Here's how the part is built. I have some questions about the finished solid (model axes, mm). Round coordinates to 2 decimals unless told otherwise and drop trailing zeros. Write each loop counter-clockwise with the first axis right and the second up, starting at its lowest first coordinate (ties: lowest second). Pieces come first, ordered by that corner, then holes. Notation, with made-up numbers: (8, 68.5) -> (18, 68.5) arc R15 ccw to (18, 88.5) -> close; hole circle Ø4 at (-35, 18.25). An arc over 180 degrees is marked (long way). Put each result on its own line as item: value. Start each with the question number.
1. We'd pull the mould along X, two halves only. Please class faces 1 (the face through (0.534, -4.065, 10.34)), 2 (the face through (-4, 2, -0.9)), 3 (the face through (4.762, 1.974, -0.844)): +X half, -X half, draft (parallel to the pull), parting line (faces both ways), or undercut.
2. I need wall thicknesses on probe 1 along Y at (x, z) = (0, 15.5); probe 2 along Y at (x, z) = (-1.25, 15.75); probe 3 along X at (y, z) = (3.5, 7.25). Which ranges of each line are inside material? Lowest first, please. Write a range as from..to.
3. For pin 1 (1 mm diameter, centred on x = 1, y = -6, fed in from +Z); pin 2 (1 mm diameter, centred on x = 4.5, z = 17, fed in from -Y); pin 3 (3 mm diameter, centred on x = 6, y = -5, fed in from -Z), each with a flat end and sliding along its axis, tell me the tip position at first contact or that it passes through.
4. Suppose I cut it at C-C (z = 7.75). Please give me the cut outline in (x, y), then the cut area to 3 significant figures.
```python
from build123d import *
from OCP.BRepFilletAPI import BRepFilletAPI_MakeChamfer

# Parameters (mm, degrees)
SKETCH1_R           = 7.5
SKETCH1_R_2         = 4.1
BOSS_EXTRUDE1_DEPTH = 21
BOSS_EXTRUDE2_START = -0.9
SKETCH2_R           = 5
SKETCH2_R_2         = 4.1
BOSS_EXTRUDE2_DEPTH = 22.8
CHAMFER1_SIZE       = 0.9
CHAMFER1_SIZE_2     = 2.472729678


with BuildPart() as part:
    # Sketch1 → Boss-Extrude1 (new body)
    with BuildSketch(Plane.XY):
        with Locations(Location((0, 0, 0), (0, 0, 180))):
            Circle(SKETCH1_R)
        with Locations(Location((0, 0, 0), (0, 0, 180))):
            Circle(SKETCH1_R_2, mode=Mode.SUBTRACT)
    extrude(amount=BOSS_EXTRUDE1_DEPTH)

    # Sketch2 → Boss-Extrude2 (add)
    with BuildSketch(Plane.XY.offset(BOSS_EXTRUDE2_START)):
        Circle(SKETCH2_R)
        with Locations(Location((0, 0, 0), (0, 0, 180))):
            Circle(SKETCH2_R_2, mode=Mode.SUBTRACT)
    extrude(amount=BOSS_EXTRUDE2_DEPTH)

    # Chamfer1
    chamfer1_edges_1 = [part.edges().sort_by_distance(p)[0] for p in [
        (-5, 0, 0),
    ]]
    chamfer1_side_1 = [part.faces().sort_by_distance(p)[0] for p in [
        (-5, 0, -0.018),
    ]]
    chamfer1_edges_2 = [part.edges().sort_by_distance(p)[0] for p in [
        (-5, 0, 21),
    ]]
    chamfer1_side_2 = [part.faces().sort_by_distance(p)[0] for p in [
        (-5.018, 0, 21),
    ]]
    chamfer1 = BRepFilletAPI_MakeChamfer(part.part.solid().wrapped)
    for e in chamfer1_edges_1:
        chamfer1.Add(CHAMFER1_SIZE - 0.0001, CHAMFER1_SIZE_2 - 0.0001, e.wrapped, chamfer1_side_1[0].wrapped)
    for e in chamfer1_edges_2:
        chamfer1.Add(CHAMFER1_SIZE_2 - 0.0001, CHAMFER1_SIZE - 0.0001, e.wrapped, chamfer1_side_2[0].wrapped)
    add(Compound.cast(chamfer1.Shape()), mode=Mode.REPLACE)  # a hair under: the kernel refuses the full size


solid = part.part
```
Verdict:
1. face 1: undercut
1. face 2: draft
1. face 3: parting line
2. probe 1: y = -7.5..-4.1, 4.1..7.5
2. probe 2: y = -7.4..-3.9, 3.9..7.4
2. probe 3: x = -6.63..-2.14, 2.14..6.63
3. pin 1: stops at z = 21.69
3. pin 2: stops at y = -6.34
3. pin 3: stops at z = -0.42
4. outline: circle Ø15 at (0, 0); hole circle Ø8.2 at (0, 0)
4. area: 124 mm^2
